from build123d import *

# Parameters (mm, degrees)
SKETCH1_R               = 140
SKETCH1_R_2             = 125
RING_DEPTH              = 12
SKETCH2_R               = 40
HUB_DEPTH               = 40
SKETCH3_W               = 16
SKETCH3_H               = 87
SPOKES_DEPTH            = 12
SKETCH4_R               = 6
BORE_DEPTH              = 40
SKETCH5_R               = 11
BEARING_SEAT_LOW_DEPTH  = 7
SKETCH6_R               = 11
BEARING_SEAT_HIGH_DEPTH = 7
SKETCH7_R               = 1.7
RING_SCREWS_DEPTH       = 12
SKETCH8_R               = 1.25
GROMMET_SCREWS_DEPTH    = 8


with BuildPart() as part:
    # Sketch1 → Ring (new body)
    with BuildSketch(Plane.XY.offset(28)):
        Circle(SKETCH1_R)
        Circle(SKETCH1_R_2, mode=Mode.SUBTRACT)
    extrude(amount=RING_DEPTH)



with BuildPart() as body_2:
    # Sketch2 → Hub (new body)
    with BuildSketch(Plane.XY):
        Circle(SKETCH2_R)
    extrude(amount=HUB_DEPTH)


with BuildPart() as part_1:
    add(part.part)

    add(body_2.part)  # Spokes merges body 2
    # Sketch3 → Spokes (add)
    with BuildSketch(Plane.XY.offset(28)):
        Polygon((39.563340091, 4.44321065), (122.305257008, 31.327689161), (117.360985098, 46.544593422), (34.619068181, 19.660114911), align=None)
        with Locations((0, 82.5)):
            Rectangle(SKETCH3_W, SKETCH3_H)
        Polygon((-34.619068181, 19.660114911), (-117.360985098, 46.544593422), (-122.305257008, 31.327689161), (-39.563340091, 4.44321065), align=None)
        Polygon((-29.395760794, -26.849380762), (-80.533077744, -97.233859273), (-67.588805834, -106.63842331), (-16.451488884, -36.253944799), align=None)
        Polygon((16.451488884, -36.253944799), (67.588805834, -106.63842331), (80.533077744, -97.233859273), (29.395760794, -26.849380762), align=None)
    extrude(amount=SPOKES_DEPTH)

    # Sketch4 → Bore (cut)
    with BuildSketch(Plane.XY):
        Circle(SKETCH4_R)
    extrude(amount=BORE_DEPTH, mode=Mode.SUBTRACT)

    # Sketch5 → Bearing_seat_low (cut)
    with BuildSketch(Plane.XY):
        Circle(SKETCH5_R)
    extrude(amount=BEARING_SEAT_LOW_DEPTH, mode=Mode.SUBTRACT)

    # Sketch6 → Bearing_seat_high (cut)
    with BuildSketch(Plane.XY.offset(33)):
        Circle(SKETCH6_R)
    extrude(amount=BEARING_SEAT_HIGH_DEPTH, mode=Mode.SUBTRACT)

    # Sketch7 → Ring_screws (cut)
    with BuildSketch(Plane.XY.offset(28)):
        with Locations((77.881545929, 107.194751755)):
            Circle(SKETCH7_R)
        with Locations((-77.881545929, 107.194751755)):
            Circle(SKETCH7_R)
        with Locations((-126.014988409, -40.944751755)):
            Circle(SKETCH7_R)
        with Locations((0, -132.5)):
            Circle(SKETCH7_R)
        with Locations((126.014988409, -40.944751755)):
            Circle(SKETCH7_R)
    extrude(amount=RING_SCREWS_DEPTH, mode=Mode.SUBTRACT)

    # Sketch8 → Grommet_screws (cut)
    with BuildSketch(Plane.XY):
        with Locations((21.213203436, 21.213203436)):
            Circle(SKETCH8_R)
        with Locations((-21.213203436, 21.213203436)):
            Circle(SKETCH8_R)
        with Locations((-21.213203436, -21.213203436)):
            Circle(SKETCH8_R)
        with Locations((21.213203436, -21.213203436)):
            Circle(SKETCH8_R)
    extrude(amount=GROMMET_SCREWS_DEPTH, mode=Mode.SUBTRACT)


solid = part_1.part
Input: part model. Units: mm. Frame: model coordinates. A direction names the side the tool comes from. Give positions to 0.01 mm unless a question says otherwise; leave off trailing zeros. Order: outer loops, then holes, each group sorted by start corner. A loop starts at its lowest first (then second) coordinate and runs counter-clockwise, first axis right, second up. Notation, with made-up numbers: (28, 22) - (37, 22) arc R29 ccw to (37, 59) - close; hole circle Ø1 at (82.5, 25). An arc over 180 degrees is marked (long way). Answer as a JSON object with one key per item and string values. Group by question number.
Q1. Cut plane A-A, the plane y = 0. Output: boundary loops of the cut face in (x, z).
Q2. Line query: probe 1 along Y at (x, z) = (0, 35); probe 2 along X at (y, z) = (0, 18); probe 3 along X at (y, z) = (-2, 33.5). Output: solid intervals per line, ascending.
Q3. Cut plane C-C, the plane y = -115. Output: boundary loops of the cut face in (x, z), then the cut area to 3 significant figures.
Q4. Mould query, pull axis Y, two halves, no side actions, for faces 4 (the face through (-1, 21, 40)), 5 (the face through (41.355, -70.531, 33.916)). Classes: pulls with the +Y half, pulls with the -Y half, needs draft (parallel to the pull), parting line crosses it, or undercut.
Q5. Set-up query: faces 1 (the face through (-72.672, 101.704, 33.916)), 2 (the face through (-2.38, -10.74, 36.45)), 3 (the face through (-32, -24, 20)). Return all of +Z, -Z, +X, -X, +Y, -Y with unobstructed straight access to the full face (end or side cutting, diameter ignored); none if empty.
Q6. Cut plane B-B, the plane z = 14.5. Output: boundary loops of the cut face in (x, y), then the cut area to 3 significant figures.
Q7. Cut plane D-D, the plane y = -75.5. Output: boundary loops of the cut face in (x, z).
Q8. First-contact query: pin 1 Ø6 at (x, z) = (17, 22.5) entering from -Y; pin 2 Ø0.8 at (x, y) = (21, 21) entering from -Z; pin 3 Ø11 at (x, y) = (-4.5, 1.5) entering from -Z. Flat tips, straight axial feed; report the tip coordinate or a pass-through.
Results:
{
 "1": {"outline": "(-140, 28) - (-125, 28) - (-125, 40) - (-140, 40) - close; (-40, 0) - (-11, 0) - (-11, 7) - (-6, 7) - (-6, 33) - (-11, 33) - (-11, 40) - (-40, 40) - close; (6, 7) - (11, 7) - (11, 0) - (40, 0) - (40, 40) - (11, 40) - (11, 33) - (6, 33) - close; (125, 28) - (140, 28) - (140, 40) - (125, 40) - close"},
 "2": {"probe 1": "-140 to -134.2, -130.8 to -125, -40 to -11, 11 to 140", "probe 2": "-40 to -6, 6 to 40", "probe 3": "-139.99 to -124.98, -39.95 to -10.82, 10.82 to 39.95, 124.98 to 139.99"},
 "3": {"outline": "(-79.84, 28) - (-48.99, 28) - (-48.99, 40) - (-79.84, 40) - close; (48.99, 28) - (79.84, 28) - (79.84, 40) - (48.99, 40) - close", "area": "740 mm^2"},
 "4": {"face 4": "needs draft", "face 5": "undercut"},
 "5": {"face 1": "+Z, -Z", "face 2": "+Z", "face 3": "-Z"},
 "6": {"outline": "circle Ø80 at (0, 0); hole circle Ø12 at (0, 0)", "area": "4,910 mm^2"},
 "7": {"outline": "(-117.9, 28) - (-99.62, 28) - (-99.62, 40) - (-117.9, 40) - close; (-64.74, 28) - (-44.97, 28) - (-44.97, 40) - (-64.74, 40) - close; (44.97, 28) - (64.74, 28) - (64.74, 40) - (44.97, 40) - close; (99.62, 28) - (117.9, 28) - (117.9, 40) - (99.62, 40) - close"},
 "8": {"pin 1": "y = -37.47", "pin 2": "z = 8", "pin 3": "z = 7"}
}
